Geometry check sheet. Reference: the model listing, model coordinates, mm. Face numbers are marked on the shaded views. A direction names the side the tool comes from. Give positions to 0.01 mm unless a question says otherwise; leave off trailing zeros. Order: outer loops, then holes, each group sorted by start corner. A loop starts at its lowest first (then second) coordinate and runs counter-clockwise, first axis right, second up.
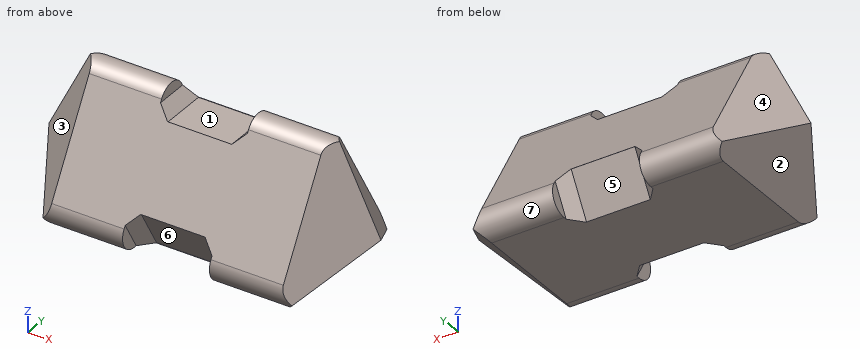
```python
from build123d import *

# Parameters (mm, degrees)
F1_DEPTH    = 20
F4_T1_DEPTH = 32.9903810568
F6_START    = 9.5
F5_W        = 7.5
F5_H        = 4
F6_DEPTH    = 10.5
F8_START    = -9.5
F7_W        = 7.5
F7_H        = 4
F8_DEPTH    = 15.5
F10_START   = -9.5
F9_W        = 7.5
F9_H        = 4
F10_DEPTH   = 10.5
F11_SIZE    = 1


# Not quite as in the source:
# - a fillet or chamfer that OpenCascade refuses, or shapes differently, is made with other operations: its cross-section is extruded or revolved along the edge and cut away or added
# - an extrude whose draft closes it to a point is written as a loft to that point


with BuildPart() as f1:
    # F0 (on Right) → F1 (new body)
    with BuildSketch(Plane.YZ):
        Polygon((-7.5, 0), (7.5, 0), (0, 12.9903810568), align=None)
    extrude(amount=F1_DEPTH)

    # F1_face (on face) → F2 section 0
    with BuildSketch(Plane(origin=(0, 0, 4.3301270189), x_dir=(0, 1, 0), z_dir=(-1, 0, 0)), mode=Mode.PRIVATE) as f2_s0:
        Polygon((7.5, 4.3301270189), (-7.5, 4.3301270189), (0, -8.6602540378), align=None)
    loft([f2_s0.sketch, Vertex(-4.3301270189, 0, 4.3301270189)], ruled=True)

    # F1_face1 (on face) → F3 section 0
    with BuildSketch(Plane(origin=(20, 0, 4.3301270189), x_dir=(0, 1, 0), z_dir=(1, 0, 0)), mode=Mode.PRIVATE) as f3_s0:
        Polygon((-7.5, -4.3301270189), (7.5, -4.3301270189), (0, 8.6602540378), align=None)
    loft([f3_s0.sketch, Vertex(24.3301270189, 0, 4.3301270189)], ruled=True)

    # F4: fillet of radius 1.5 on 3 edges, made by hand

    # F4_s2 → F4_t1 (cut)
    with BuildSketch(Plane.YZ.offset(-6.4951905284)):
        with BuildLine():
            ThreePointArc((-1.2990381057, 10.7403810568), (0, 11.4903810568), (1.2990381057, 10.7403810568))
            Line((1.2990381057, 10.7403810568), (0, 12.9903810568))
            Line((0, 12.9903810568), (-1.2990381057, 10.7403810568))
        make_face()
        with BuildLine():
            ThreePointArc((-4.9019237886, 0), (-6.2009618943, 0.75), (-6.2009618943, 2.25))
            Line((-6.2009618943, 2.25), (-7.5, 0))
            Line((-7.5, 0), (-4.9019237886, 0))
        make_face()
        with BuildLine():
            ThreePointArc((4.9019237886, 0), (6.2009618943, 0.75), (6.2009618943, 2.25))
            Line((6.2009618943, 2.25), (7.5, 0))
            Line((7.5, 0), (4.9019237886, 0))
        make_face()
    extrude(amount=F4_T1_DEPTH, mode=Mode.SUBTRACT)

    # F5 (on Top) → F6 (cut)
    with BuildSketch(Plane.XY.offset(F6_START)):
        with Locations((10, -0.0009618943)):
            Rectangle(F5_W, F5_H)
    extrude(amount=F6_DEPTH, mode=Mode.SUBTRACT)

    # F7 (on face) → F8 (cut)
    with BuildSketch(Plane(origin=(0, -5.625, 3.2475952642), x_dir=(1, 0, 0), z_dir=(0, -0.8660254038, 0.5)).offset(F8_START)):
        with Locations((10, 3.7480762114)):
            Rectangle(F7_W, F7_H)
    extrude(amount=-F8_DEPTH, mode=Mode.SUBTRACT)

    # F9 (on face) → F10 (cut)
    with BuildSketch(Plane(origin=(0, 5.625, 3.2475952642), x_dir=(-1, 0, 0), z_dir=(0, 0.8660254038, 0.5)).offset(F10_START)):
        with Locations((-10, 3.7519237886)):
            Rectangle(F9_W, F9_H)
    extrude(amount=-F10_DEPTH, mode=Mode.SUBTRACT)

    # F11
    f11_edges = [f1.edges().sort_by_distance(p)[0] for p in [
        (6.25, 4.476279, 1.743524),
        (13.75, 4.476279, 1.743524),
        (6.25, -4.478203, 1.746857),
        (13.75, -4.478203, 1.746857),
        (6.25, -0.000962, 9.5),
        (13.75, -0.000962, 9.5),
    ]]
    chamfer(f11_edges, length=F11_SIZE)


solid = f1.part
```
Q1. Cross-section at C-C, the plane y = -4.25. Record the boundary of the cut face in (x, z), and give its area (3 significant figures).
Q2. Gauge pin test, flat ends, axial feed: P1, Ø6, axis at y = -3, z = 8, coming from the -X side; P2, Ø2, axis at x = 13, z = 6.5, coming from the +Y side; P3, Ø0.9, axis at y = -5, z = 1, coming from the -X side. Record the tip position at first contact, or that the pin passes through.
Q3. Release check for a two-part mould opening along Y. For the marked faces 1, 2, 3 and 4 record: pulls with the +Y half, pulls with the -Y half, needs draft (parallel to the pull), parting line crosses it, or undercut.
Q4. Thickness scan on L1, parallel to Y at x = 14.75, z = 2.5; L2, parallel to Y at x = 1, z = 10.75; L3, parallel to Z at x = 16, y = 5. Record the ranges inside material, lowest first.
Q5. Cross-section at B-B, the plane z = 1.25. Record the boundary of the cut face in (x, y).
Q6. Cross-section at D-D, the plane x = 16.5. Record the boundary of the cut face in (y, z), and give its area (3 significant figures).
Q7. Access from +Z, -Z, +X, -X, +Y, -Y to the whole of each face (thin tool, end or side, straight path). Record for the marked faces 5, 6 and 7.
Answers follow:
1. outline: (-1.88, 1.88) - (0, 0) - (6.57, 0) - (7.25, 1.35) - (12.75, 1.35) - (13.43, 0) - (20, 0) - (21.88, 1.88) - (20, 5.63) - (0, 5.63) - close
1. area: 115 mm2
2. P1: stops at x = -2.9
2. P2: stops at y = 4.32
2. P3: stops at x = -1.45
3. face 1: undercut
3. face 2: needs draft
3. face 3: pulls with the -Y half
3. face 4: pulls with the +Y half
4. L1: y = -6.06 to 6.06
4. L2: y = -1.29 to 1.29
4. L3: z = 0 to 4.33
5. outline: (-1.25, -5.33) - (-0.34, -6.38) - (6.25, -6.38) - (6.25, -5.35) - (7.25, -4.19) - (12.75, -4.19) - (13.75, -5.35) - (13.75, -6.38) - (20.34, -6.38) - (21.25, -5.33) - (21.25, 5.33) - (20.34, 6.38) - (13.75, 6.38) - (13.75, 5.35) - (12.75, 4.19) - (7.25, 4.19) - (6.25, 5.35) - (6.25, 6.38) - (-0.34, 6.38) - (-1.25, 5.33) - close
6. outline: (-6.2, 2.25) arc R1.5 ccw to (-4.9, 0) - (4.9, 0) arc R1.5 ccw to (6.2, 2.25) - (1.3, 10.74) arc R1.5 ccw to (-1.3, 10.74) - close
6. area: 92.8 mm2
7. face 5: -Z, +Y
7. face 6: -Z, -Y
7. face 7: +X, -X, +Y
